Part print with two shaded views. Sizes in mm from the minimum x, y, z corner. Coordinates: 2 decimals unless noted, no trailing zeros. Order: outer loops, then holes, each group sorted by start corner. A loop starts at its lowest first (then second) coordinate and runs counter-clockwise, first axis right, second up.
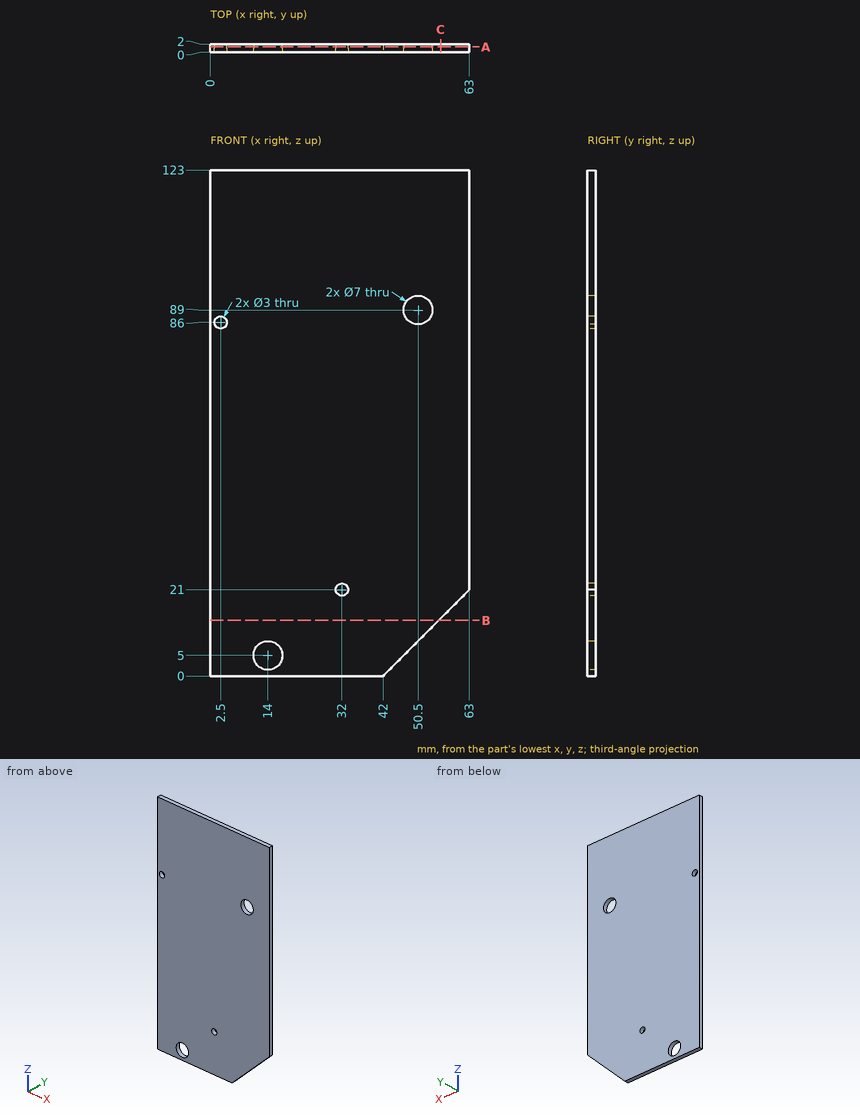
Q1. Wall check: line 1 along Z through (x, y) = (32, 0.65); line 2 along X through (y, z) = (0.85, 89); line 3 along Z through (x, y) = (50.5, 1.2). Give the ranges that are in metal, low to high.
Results list:
line 1: z = 0 to 19.5, 22.5 to 123
line 2: x = 0 to 47, 54 to 63
line 3: z = 8.5 to 85.5, 92.5 to 123
Q2. Cut at A-A on y = 1.3. Write the cut outline in (x, z).
Results list:
outline: (0, 0) - (42, 0) - (63, 21) - (63, 123) - (0, 123) - close; hole circle Ø3 at (2.5, 86); hole circle Ø7 at (14, 5); hole circle Ø3 at (32, 21); hole circle Ø7 at (50.5, 89)
Q3. Cut at C-C on x = 56. Write the cut outline in (y, z).
Results list:
outline: (0, 14) - (2, 14) - (2, 123) - (0, 123) - close
Q4. Cut at B-B on z = 13.5. Write the cut outline in (x, y).
Results list:
outline: (0, 0) - (55.5, 0) - (55.5, 2) - (0, 2) - close
